```python
from build123d import *

# Parameters (mm, degrees)
SKETCH_1_W          = 108
SKETCH_1_H          = 30
EXTRUDE_1_DEPTH     = 12
SKETCH_2_W          = 5
SKETCH_2_H          = 12
CUT_EXTRUDE_1_DEPTH = 8
SKETCH_3_W          = 0.8
SKETCH_3_H          = 10
EXTRUDE_2_DEPTH     = 6
SKETCH_4_W          = 11
SKETCH_4_H          = 5
CUT_EXTRUDE_2_DEPTH = 8
SKETCH_5_W          = 10
SKETCH_5_H          = 0.8
EXTRUDE_3_DEPTH     = 6
SKETCH_6_W          = 11
SKETCH_6_H          = 5
CUT_EXTRUDE_3_DEPTH = 8
SKETCH_7_W          = 10
SKETCH_7_H          = 0.8
EXTRUDE_4_DEPTH     = 6
SKETCH_8_W          = 11
SKETCH_8_H          = 5
CUT_EXTRUDE_4_DEPTH = 8
SKETCH_9_W          = 10
SKETCH_9_H          = 0.8
EXTRUDE_5_DEPTH     = 6
FILLET_1_R          = 5
FILLET_2_R          = 8


with BuildPart() as part:
    # 草图1 → 凸台-拉伸1 (new body)
    with BuildSketch(Plane(origin=(0, 0, 0), x_dir=(-1, 0, 0), z_dir=(0, 0, -1))):
        Rectangle(SKETCH_1_W, SKETCH_1_H)
    extrude(amount=-EXTRUDE_1_DEPTH)

    # 草图2 → 切除-拉伸1 (cut)
    with BuildSketch(Plane.ZY.offset(54)):
        with Locations((6, 4)):
            Rectangle(SKETCH_2_W, SKETCH_2_H)
    extrude(amount=-CUT_EXTRUDE_1_DEPTH, mode=Mode.SUBTRACT)

    # 草图3 → 凸台-拉伸2 (add)
    with BuildSketch(Plane.ZY.offset(46)):
        with Locations((7.7, 4)):
            Rectangle(SKETCH_3_W, SKETCH_3_H)
    extrude(amount=EXTRUDE_2_DEPTH)

    # 草图4 → 切除-拉伸2 (cut)
    with BuildSketch(Plane.XZ.offset(15)):
        with Locations((-34.5, 6)):
            Rectangle(SKETCH_4_W, SKETCH_4_H)
    extrude(amount=-CUT_EXTRUDE_2_DEPTH, mode=Mode.SUBTRACT)

    # 草图5 → 凸台-拉伸3 (add)
    with BuildSketch(Plane.XZ.offset(7)):
        with Locations((-34.5, 7.8)):
            Rectangle(SKETCH_5_W, SKETCH_5_H)
    extrude(amount=EXTRUDE_3_DEPTH)

    # 草图6 → 切除-拉伸3 (cut)
    with BuildSketch(Plane.XZ.offset(15)):
        with Locations((-3.5, 6)):
            Rectangle(SKETCH_6_W, SKETCH_6_H)
    extrude(amount=-CUT_EXTRUDE_3_DEPTH, mode=Mode.SUBTRACT)

    # 草图7 → 凸台-拉伸4 (add)
    with BuildSketch(Plane.XZ.offset(7)):
        with Locations((-3.5, 7.8)):
            Rectangle(SKETCH_7_W, SKETCH_7_H)
    extrude(amount=EXTRUDE_4_DEPTH)

    # 草图8 → 切除-拉伸4 (cut)
    with BuildSketch(Plane.XZ.offset(15)):
        with Locations((17.5, 6)):
            Rectangle(SKETCH_8_W, SKETCH_8_H)
    extrude(amount=-CUT_EXTRUDE_4_DEPTH, mode=Mode.SUBTRACT)

    # 草图9 → 凸台-拉伸5 (add)
    with BuildSketch(Plane.XZ.offset(7)):
        with Locations((17.5, 7.8)):
            Rectangle(SKETCH_9_W, SKETCH_9_H)
    extrude(amount=EXTRUDE_5_DEPTH)

    # 草图10 → 旋转1 (revolve)
    with BuildSketch(Plane.XY.offset(4.899865492)):
        Polygon((54, 4.5), (54, 1.5), (69, 1.5), (69, 3.5), (59, 3.5), (59, 4.5), align=None)
    revolve(axis=Axis((54, 1.5, 4.899865492), (1, 0, 0)))

    # 圆角1
    fillet_1_edges = [part.edges().sort_by_distance(p)[0] for p in [
        (0, 15, 12),
        (0, 15, 0),
    ]]
    fillet(fillet_1_edges, radius=FILLET_1_R)

    # 圆角2
    fillet_2_edges = [part.edges().sort_by_distance(p)[0] for p in [
        (-54, -15, 6),
        (54, -15, 6),
    ]]
    fillet(fillet_2_edges, radius=FILLET_2_R)


solid = part.part
```
The model under review builds one solid part; all positions refer to its coordinate system, in mm. A direction names the side the tool comes from. Round coordinates to 2 decimals unless told otherwise and drop trailing zeros. Loops run counter-clockwise (first coordinate to the right, second up) from the corner with the lowest first, then second, coordinate; pieces in that order, holes last. Notation, with made-up numbers: M 85.5,-33.75 L 140.5,-33.75 A22 ccw 140.5,-2.75 Z; hole C 15.5,-27.75 d7. An arc over 180 degrees is marked long. Answer as a JSON object with one key per item and string values.
(1) Take a section at B-B on x = -7. Give the boundary of the cut face in (y, z), and give its area (3 significant figures).
Resolved:
{"outline": "M -15,0 L 10,0 A5 ccw 15,5 L 15,7 A5 ccw 10,12 L -15,12 L -15,8.5 L -7,8.5 L -7,8.2 L -13,8.2 L -13,7.4 L -7,7.4 L -7,3.5 L -15,3.5 Z", "area": "314 mm²"}
(2) Draft analysis for pull direction X (two halves, no side actions). For faces 1 (the cylindrical face through (56.46, 0.85, 1.97)), 2 (the flat face through (59, 2, 7)), 3 (the cylindrical face through (-51.594, -12.719, 6.084)), 4 (the flat face through (17, -11, 3.5)), state which applies: released by +X, released by -X, zero draft, split by the parting line, or undercut.
Resolved:
{"face 1": "zero draft", "face 2": "released by +X", "face 3": "released by -X", "face 4": "undercut"}
(3) Take a section at A-A on y = -10.25. Give the boundary of the cut face in (x, z).
Resolved:
{"outline": "M -53.31,0 L 53.31,0 L 53.31,12 L -53.31,12 Z; M -39.5,7.4 L -29.5,7.4 L -29.5,8.2 L -39.5,8.2 Z; M -8.5,7.4 L 1.5,7.4 L 1.5,8.2 L -8.5,8.2 Z; M 12.5,7.4 L 22.5,7.4 L 22.5,8.2 L 12.5,8.2 Z; hole M -40,3.5 L -29,3.5 L -29,8.5 L -40,8.5 Z; hole M -9,3.5 L 2,3.5 L 2,8.5 L -9,8.5 Z; hole M 12,3.5 L 23,3.5 L 23,8.5 L 12,8.5 Z"}
(4) Tool access review of faces 5 (the flat face through (1, 15, 6)), 6 (the flat face through (23, -11, 6)): name each direction out of +Z, -Z, +X, -X, +Y, -Y from which nothing blocks a thin tool from reaching the whole face with its end or side.
Resolved:
{"face 5": "+Z, -Z, +X, -X, +Y", "face 6": "-Y"}
(5) Take a section at C-C on y = 1.5. Give the boundary of the cut face in (x, z).
Resolved:
{"outline": "M -54,0 L 54,0 L 54,1.9 L 59,1.9 L 59,2.9 L 69,2.9 L 69,6.9 L 59,6.9 L 59,7.9 L 54,7.9 L 54,12 L -54,12 L -54,8.5 L -46,8.5 L -46,8.1 L -52,8.1 L -52,7.3 L -46,7.3 L -46,3.5 L -54,3.5 Z"}
(6) To check wall thickness, follow line 1 along Z through (x, y) = (18.5, -9.5); line 2 along X through (y, z) = (9.25, 6); line 3 along X through (y, z) = (1.75, 10.75). State the ranges of each line that lie inside material, in increasing order.
Resolved:
{"line 1": "0 to 3.5, 7.4 to 8.2, 8.5 to 12", "line 2": "-46 to 54", "line 3": "-54 to 54"}
(7) Clearance check with flat-ended pins moving along their axes: P1, Ø4, axis at y = -9.5, z = 5, coming from the -X side; P2, Ø0.9, axis at x = -4, z = 7.5, coming from the -Y side; P3, Ø1.5, axis at x = 18.5, z = 5.5, coming from the -Y side. State where each tip first meets the part, or that it passes through.
Resolved:
{"P1": "x = -53.98", "P2": "y = -13", "P3": "y = -7"}
(8) Take a section at D-D on x = 34. Give the boundary of the cut face in (y, z).
Resolved:
{"outline": "M -15,0 L 10,0 A5 ccw 15,5 L 15,7 A5 ccw 10,12 L -15,12 Z"}
